from build123d import *

# Parameters (mm, degrees)
SKETCH_1_W          = 58
SKETCH_1_H          = 50
EXTRUDE_1_DEPTH     = 10
SKETCH_2_R          = 29
SKETCH_2_R_2        = 26.1
EXTRUDE_2_DEPTH     = 7.5
SKETCH_3_R          = 26.1
SKETCH_3_R_2        = 24
EXTRUDE_3_DEPTH     = 0.5
SKETCH_4_W          = 6
SKETCH_4_H          = 5
EXTRUDE_4_DEPTH     = 8
CUT_EXTRUDE_1_REACH = 12
SKETCH_5_R          = 1.55
SKETCH_6_R          = 3
CUT_EXTRUDE_2_DEPTH = 3
SKETCH_7_R          = 15
CUT_EXTRUDE_3_DEPTH = 11


with BuildPart() as part:
    # 草图1 → 凸台-拉伸1 (new body)
    with BuildSketch(Plane.XY):
        with BuildLine():
            ThreePointArc((-29, 25), (0, 54), (29, 25))
            Line((29, 25), (-29, 25))
        make_face()
        Rectangle(SKETCH_1_W, SKETCH_1_H)
    extrude(amount=EXTRUDE_1_DEPTH)

    # 草图2 → 凸台-拉伸2 (add)
    with BuildSketch(Plane(origin=(0, 0, 0), x_dir=(-1, 0, 0), z_dir=(0, 0, -1))):
        with Locations((0, 25)):
            Circle(SKETCH_2_R)
        with Locations((0, 25)):
            Circle(SKETCH_2_R_2, mode=Mode.SUBTRACT)
    extrude(amount=EXTRUDE_2_DEPTH)

    # 草图3 → 凸台-拉伸3 (add)
    with BuildSketch(Plane(origin=(0, 0, 0), x_dir=(-1, 0, 0), z_dir=(0, 0, -1))):
        with Locations((0, 25)):
            Circle(SKETCH_3_R)
        with Locations((0, 25)):
            Circle(SKETCH_3_R_2, mode=Mode.SUBTRACT)
    extrude(amount=EXTRUDE_3_DEPTH)

    # 草图4 → 凸台-拉伸4 (add)
    with BuildSketch(Plane(origin=(0, 0, 0), x_dir=(-1, 0, 0), z_dir=(0, 0, -1))):
        with Locations((-26, -17.5)):
            Rectangle(SKETCH_4_W, SKETCH_4_H)
        with Locations((-26, -22.5)):
            Rectangle(SKETCH_4_W, SKETCH_4_H)
        with Locations((26, -17.5)):
            Rectangle(SKETCH_4_W, SKETCH_4_H)
        with Locations((26, -22.5)):
            Rectangle(SKETCH_4_W, SKETCH_4_H)
    extrude(amount=EXTRUDE_4_DEPTH)

    # 草图5 → 切除-拉伸1 (cut, up to next)
    with BuildSketch(Plane(origin=(0, 0, 0), x_dir=(-1, 0, 0), z_dir=(0, 0, -1)), mode=Mode.PRIVATE) as cut_extrude_1_sk1:
        with Locations((-19, -20)):
            Circle(SKETCH_5_R)
    cut_extrude_1_tool1 = extrude(cut_extrude_1_sk1.sketch, amount=-CUT_EXTRUDE_1_REACH, mode=Mode.PRIVATE) & part.part
    add(cut_extrude_1_tool1.solids().sort_by_distance((19, -20, 0))[0], mode=Mode.SUBTRACT)
    # 草图5 → 切除-拉伸1 (cut, up to next)
    with BuildSketch(Plane(origin=(0, 0, 0), x_dir=(-1, 0, 0), z_dir=(0, 0, -1)), mode=Mode.PRIVATE) as cut_extrude_1_sk2:
        with Locations((-9, -20)):
            Circle(SKETCH_5_R)
    cut_extrude_1_tool2 = extrude(cut_extrude_1_sk2.sketch, amount=-CUT_EXTRUDE_1_REACH, mode=Mode.PRIVATE) & part.part
    add(cut_extrude_1_tool2.solids().sort_by_distance((9, -20, 0))[0], mode=Mode.SUBTRACT)
    # 草图5 → 切除-拉伸1 (cut, up to next)
    with BuildSketch(Plane(origin=(0, 0, 0), x_dir=(-1, 0, 0), z_dir=(0, 0, -1)), mode=Mode.PRIVATE) as cut_extrude_1_sk3:
        with Locations((9, -20)):
            Circle(SKETCH_5_R)
    cut_extrude_1_tool3 = extrude(cut_extrude_1_sk3.sketch, amount=-CUT_EXTRUDE_1_REACH, mode=Mode.PRIVATE) & part.part
    add(cut_extrude_1_tool3.solids().sort_by_distance((-9, -20, 0))[0], mode=Mode.SUBTRACT)
    # 草图5 → 切除-拉伸1 (cut, up to next)
    with BuildSketch(Plane(origin=(0, 0, 0), x_dir=(-1, 0, 0), z_dir=(0, 0, -1)), mode=Mode.PRIVATE) as cut_extrude_1_sk4:
        with Locations((19, -20)):
            Circle(SKETCH_5_R)
    cut_extrude_1_tool4 = extrude(cut_extrude_1_sk4.sketch, amount=-CUT_EXTRUDE_1_REACH, mode=Mode.PRIVATE) & part.part
    add(cut_extrude_1_tool4.solids().sort_by_distance((-19, -20, 0))[0], mode=Mode.SUBTRACT)

    # 草图6 → 切除-拉伸2 (cut)
    with BuildSketch(Plane.XY.offset(10)):
        with Locations((19, -20)):
            Circle(SKETCH_6_R)
        with Locations((9, -20)):
            Circle(SKETCH_6_R)
        with Locations((-9, -20)):
            Circle(SKETCH_6_R)
        with Locations((-19, -20)):
            Circle(SKETCH_6_R)
    extrude(amount=-CUT_EXTRUDE_2_DEPTH, mode=Mode.SUBTRACT)

    # 草图7 → 切除-拉伸3 (cut, through all)
    with BuildSketch(Plane(origin=(0, 0, 0), x_dir=(-1, 0, 0), z_dir=(0, 0, -1))):
        with Locations((0, 25)):
            Circle(SKETCH_7_R)
    extrude(amount=-CUT_EXTRUDE_3_DEPTH, mode=Mode.SUBTRACT)


solid = part.part
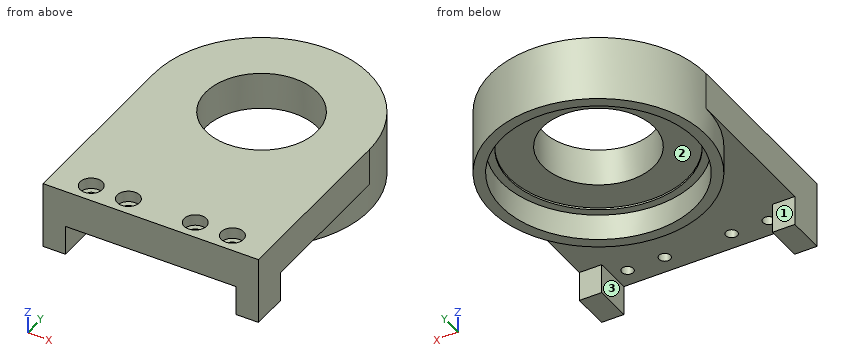
Here's how the part is built. I have some questions about the finished solid (model axes, mm). Face numbers are marked on the shaded views. A direction names the side the tool comes from. Coordinates: 2 decimals unless noted, no trailing zeros. Loops run counter-clockwise (first coordinate to the right, second up) from the corner with the lowest first, then second, coordinate; pieces in that order, holes last.
1. For P1, Ø2, axis at y = 14, z = -1.5, coming from the -X side; P2, Ø7, axis at x = 9, y = -20, coming from the -Z side; P3, Ø4, axis at x = 19, y = -20, coming from the +Z side, each with a flat end and sliding along its axis, tell me the tip position at first contact or that it passes through.
2. I need wall thicknesses on L1, parallel to Y at x = 9, z = 2; L2, parallel to Y at x = 0, z = -3.25; L3, parallel to Y at x = -9, z = 8.1. Which ranges of each line are inside material? Lowest first, please.
3. Imagine slicing it at D-D, the plane x = -8.5. Please give me the cut outline in (y, z), and give its area (3 significant figures).
4. Imagine slicing it at A-A, the plane x = 13.5. Please give me the cut outline in (y, z), and give its area (3 significant figures).
5. Imagine slicing it at B-B, the plane y = -20. Count the separate pieces of the cut face and the enclosed holes in it, and give its area (3 significant figures).
6. For the marked faces 1, 2 and 3, which set-ups out of +Z, -Z, +X, -X, +Y, -Y let a thin tool reach every point of the face, with its end or its side?
7. Imagine slicing it at C-C, the plane y = 12.5. Please give me the cut outline in (x, z), and give its area (3 significant figures).
Taken from the geometry:
1. P1: stops at x = -27.22
1. P2: stops at z = 0
1. P3: stops at z = 7
2. L1: y = -25 to -21.55, -18.45 to 13, 37 to 52.57
2. L2: y = -4 to -1.1, 51.1 to 54
2. L3: y = -25 to -23, -17 to 13, 37 to 52.57
3. outline: (-25, 0) - (-21.47, 0) - (-21.47, 7) - (-22.96, 7) - (-22.96, 10) - (-25, 10) - close; (-18.53, 0) - (-2.73, 0) - (-2.73, -7.5) - (0.32, -7.5) - (0.32, -0.5) - (2.56, -0.5) - (2.56, 0) - (12.64, 0) - (12.64, 10) - (-17.04, 10) - (-17.04, 7) - (-18.53, 7) - close; (37.36, 0) - (47.44, 0) - (47.44, -0.5) - (49.68, -0.5) - (49.68, -7.5) - (52.73, -7.5) - (52.73, 10) - (37.36, 10) - close
3. area: 540 mm2
4. outline: (-25, 0) - (-0.67, 0) - (-0.67, -7.5) - (2.66, -7.5) - (2.66, -0.5) - (5.16, -0.5) - (5.16, 0) - (18.46, 0) - (18.46, 10) - (-25, 10) - close; (31.54, 0) - (44.84, 0) - (44.84, -0.5) - (47.34, -0.5) - (47.34, -7.5) - (50.67, -7.5) - (50.67, 10) - (31.54, 10) - close
4. area: 678 mm2
5. separate pieces: 5
5. enclosed holes: 0
5. area: 517 mm2
6. face 1: -Z, +X, -X
6. face 2: -Z
6. face 3: -Z, -Y
7. outline: (-29, 0) - (-26.17, 0) - (-26.17, -7.5) - (-22.91, -7.5) - (-22.91, -0.5) - (-20.49, -0.5) - (-20.49, 0) - (-8.29, 0) - (-8.29, 10) - (-29, 10) - close; (8.29, 0) - (20.49, 0) - (20.49, -0.5) - (22.91, -0.5) - (22.91, -7.5) - (26.17, -7.5) - (26.17, 0) - (29, 0) - (29, 10) - (8.29, 10) - close
7. area: 465 mm2
